Print and shaded views of the part. All mm, measured from the part's lowest x, y and z. A direction names the side the tool comes from. Give positions to 0.01 mm unless a question says otherwise; leave off trailing zeros. Loops run counter-clockwise (first coordinate to the right, second up) from the corner with the lowest first, then second, coordinate; pieces in that order, holes last. Notation, with made-up numbers: M 68,50.25 L 78,50.25 A7 cw 78,55.25 Z; hole C -34,45.25 d2. An arc over 180 degrees is marked long. Answer as CSV lines item,"result".
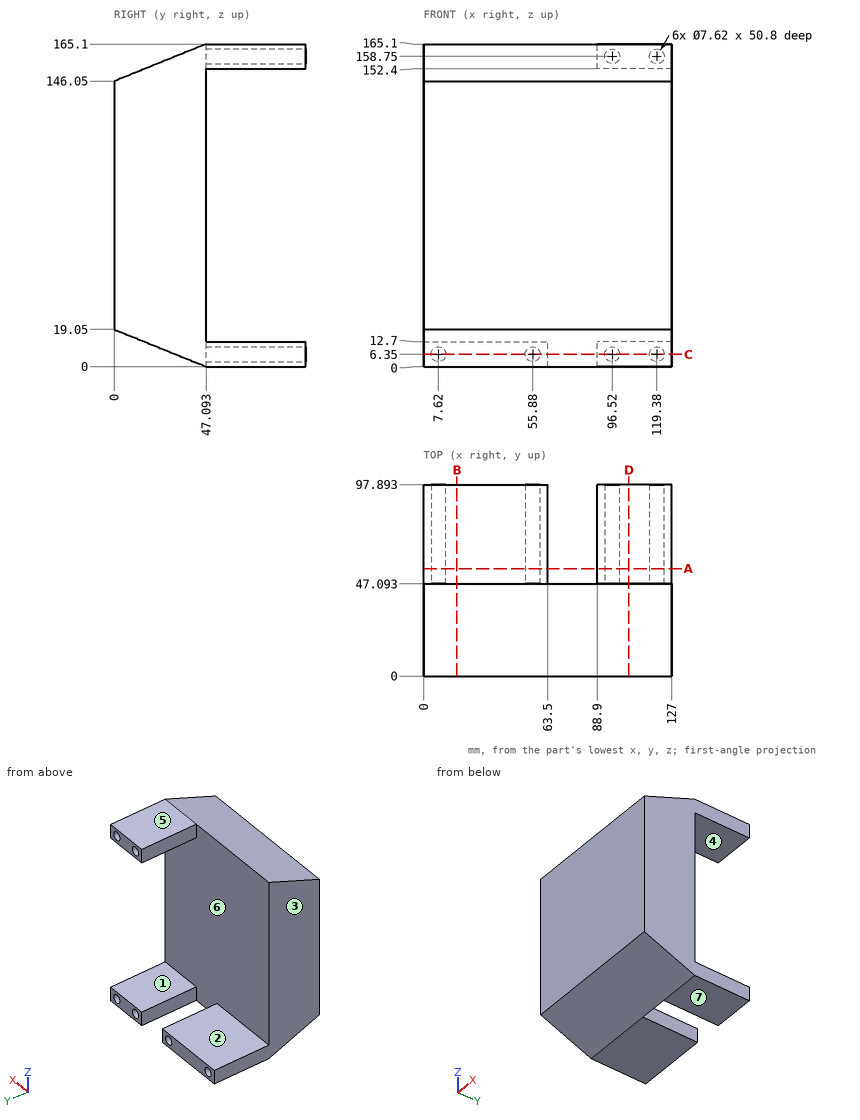
Q1. Wall check: line 1 (Z direction, x = 119, y = 61); line 2 (Z direction, x = 119.38, y = 83); line 3 (Z direction, x = 7.62, y = 65). Give the ranges that are in metal, low to high. Write a range as [from, to].
Solution:
line 1,"z = [0, 2.56], [10.14, 12.7], [152.4, 154.96], [162.54, 165.1]"
line 2,"z = [0, 2.54], [10.16, 12.7], [152.4, 154.94], [162.56, 165.1]"
line 3,"z = [0, 2.54], [10.16, 12.7]"
Q2. Cut at A-A (y = 55). Give the number of separate pieces and of enclosed holes in the cut face, and give its area (3 significant figures).
Solution:
separate pieces,"3"
enclosed holes,"6"
area,"1,500 mm²"
Q3. Cut at B-B (x = 17). Write the cut outline in (y, z).
Solution:
outline,"M 0,19.05 L 47.09,0 L 97.89,0 L 97.89,12.7 L 47.09,12.7 L 47.09,165.1 L 0,146.05 Z"
Q4. Mould opens along Z. For the marked faces 4, 5, 6 and 7 say: released by +Z, released by -Z, zero draft, split by the parting line, or undercut.
Solution:
face 4,"undercut"
face 5,"released by +Z"
face 6,"undercut"
face 7,"released by -Z"
Q5. Pin check, flat tips, straight feed: P1, Ø4.5, axis at x = 7.62, z = 6.35, coming from the -Y side; P2, Ø4.5, axis at x = 119.38, z = 6.35, coming from the +Y side; P3, Ø6.5, axis at y = 66.5, z = 161.5, coming from the -X side. Stop position of each tip, or through.
Solution:
P1,"stops at y = 25.83"
P2,"stops at y = 47.09"
P3,"stops at x = 88.9"
Q6. Cut at D-D (x = 105). Write the cut outline in (y, z), and give its area (3 significant figures).
Solution:
outline,"M 0,19.05 L 47.09,0 L 97.89,0 L 97.89,12.7 L 47.09,12.7 L 47.09,152.4 L 97.89,152.4 L 97.89,165.1 L 47.09,165.1 L 0,146.05 Z"
area,"8,170 mm²"
Q7. Cut at C-C (z = 6.35). Write the cut outline in (x, y) (1 decimal).
Solution:
outline,"M 0,31.4 L 127,31.4 L 127,97.9 L 123.2,97.9 L 123.2,47.1 L 115.6,47.1 L 115.6,97.9 L 100.3,97.9 L 100.3,47.1 L 92.7,47.1 L 92.7,97.9 L 88.9,97.9 L 88.9,47.1 L 63.5,47.1 L 63.5,97.9 L 59.7,97.9 L 59.7,47.1 L 52.1,47.1 L 52.1,97.9 L 11.4,97.9 L 11.4,47.1 L 3.8,47.1 L 3.8,97.9 L 0,97.9 Z"
Q8. Which spindle directions (+Z, -Z, +X, -X, +Y, -Y) get a long thin tool onto all of the face, cutting with end or side? Do the marked faces 1, 2 and 3. Say none if no direction does.
Solution:
face 1,"+X, -X, +Y"
face 2,"+Z, +X, -X, +Y"
face 3,"+Z, -Z, -X, +Y, -Y"
